Build history of the part. All positions in model axes, mm. A direction names the side the tool comes from. Coordinates: 2 decimals unless noted, no trailing zeros. Loops run counter-clockwise (first coordinate to the right, second up) from the corner with the lowest first, then second, coordinate; pieces in that order, holes last.
Item 1: 3-axis set-ups, long thin cutter, end or side, ignore diameter. For faces 4 (the face through (50.076, 15.77, 10.14)), 5 (the face through (-36, 12, 50)): which of +Z, -Z, +X, -X, +Y, -Y reach the whole face in a straight line?
Item 2: Mould opens along X. For faces 1 (the face through (36, 12, 0)), 2 (the face through (-4.88, 37.18, 24.65)), 3 (the face through (50.076, 15.77, 40.14)) say: released by +X, released by -X, zero draft, split by the parting line, or undercut.
Item 3: Flat gauge pins, fed straight in: pin 1 (1.5 mm diameter, centred on x = -12.5, z = 37, fed in from -Y); pin 2 (5 mm diameter, centred on x = 2, z = 28, fed in from +Y); pin 3 (8 mm diameter, centred on y = 15, z = 44, fed in from -X); pin 4 (12 mm diameter, centred on x = 9, y = -24.5, fed in from -Z). Where does each tip first touch, or does it go through?
Item 4: Drill centre lines: line 1 along Y through (x, z) = (0, 36); line 2 along Y through (x, z) = (-7.5, 38); line 3 along X through (y, z) = (2, 8). Where is each one in solid material? Low to high.
Item 5: Cut at A-A (z = 32.5). List the corners of the cut face in (x, y), and give its area (3 significant figures).
from build123d import *


with BuildPart() as f1:
    # F0 (on Front) → F1 (revolve)
    with BuildSketch(Plane.XZ):
        with BuildLine():
            Line((37.5, 50), (37.5, 0))
            Line((37.5, 0), (52.5, 0))
            Line((52.5, 0), (52.5, 20))
            ThreePointArc((52.5, 20), (47.5, 25), (52.5, 30))
            Line((52.5, 30), (52.5, 50))
            Line((52.5, 50), (37.5, 50))
        make_face()
        with BuildLine():
            ThreePointArc((52.5, 30), (47.5, 25), (52.5, 20))
            Line((52.5, 20), (52.5, 30))
        make_face()
        with BuildLine():
            Line((52.5, 30), (52.5, 20))
            ThreePointArc((52.5, 20), (56.0355339059, 21.4644660941), (57.5, 25))
            ThreePointArc((57.5, 25), (56.0355339059, 28.5355339059), (52.5, 30))
        make_face()
    revolve(axis=Axis((0, 0, 25), (0, 0, 1)))


solid = f1.part
Filled sheet:
1. face 4: -Z
1. face 5: +Z, +X, -X, +Y, -Y
2. face 1: zero draft
2. face 2: undercut
2. face 3: split by the parting line
3. pin 1: stops at y = -51.17
3. pin 2: stops at y = 57.45
3. pin 3: stops at x = -51.33
3. pin 4: passes through
4. line 1: y = -52.5 to -37.5, 37.5 to 52.5
4. line 2: y = -51.96 to -36.74, 36.74 to 51.96
4. line 3: x = -52.46 to -37.45, 37.45 to 52.46
5. outline: circle Ø105 at (0, 0); hole circle Ø75 at (0, 0)
5. area: 4,240 mm2
